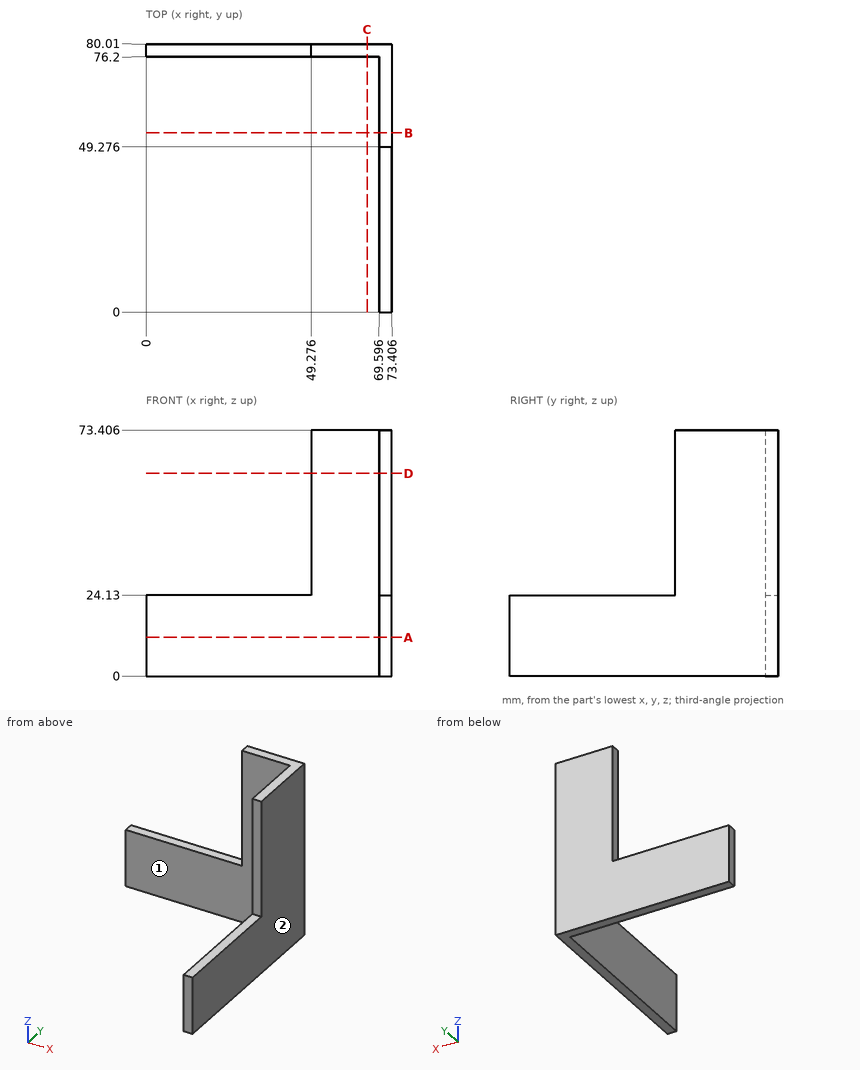
Can you work these out from the drawing? Everything is in mm from the part's minimum corner. A direction names the side the tool comes from. Coordinates: 2 decimals unless noted, no trailing zeros. Loops run counter-clockwise (first coordinate to the right, second up) from the corner with the lowest first, then second, coordinate; pieces in that order, holes last.
1) Will these pins go through, and if not, where does the flat tip stop? pin 1 Ø1.1 at (x, z) = (71.5, 37) entering from -Y; pin 2 Ø1.9 at (x, y) = (28, 78.5) entering from +Z; pin 3 Ø4 at (y, z) = (8.5, 17.5) entering from -X.
Reported:
pin 1: stops at y = 49.28
pin 2: stops at z = 24.13
pin 3: stops at x = 69.6
2) Imagine slicing it at C-C (x = 66). List the corners of the cut face in (y, z) for me, and give its area (3 significant figures).
Reported:
outline: (76.2, 0) - (80.01, 0) - (80.01, 73.41) - (76.2, 73.41) - close
area: 280 mm2
3) Imagine slicing it at B-B (y = 53.5). List the corners of the cut face in (x, z) for me.
Reported:
outline: (69.6, 0) - (73.41, 0) - (73.41, 73.41) - (69.6, 73.41) - close
4) Which directions (+Z, -Z, +X, -X, +Y, -Y) give clear straight access to the entire face, cutting with the end or side of a thin tool? Please do the marked faces 1 and 2.
Reported:
face 1: +Z, -Z, -X, -Y
face 2: +Z, -Z, +X, +Y, -Y
5) Imagine slicing it at A-A (z = 11.5). List the corners of the cut face in (x, y) for me, and give its area (3 significant figures).
Reported:
outline: (0, 76.2) - (69.6, 76.2) - (69.6, 0) - (73.41, 0) - (73.41, 80.01) - (0, 80.01) - close
area: 570 mm2
6) Please list where these lines run through material, in increasing order: line 1 along X through (y, z) = (56.5, 69.5); line 2 along Y through (x, z) = (36.5, 3).
Reported:
line 1: x = 69.6 to 73.41
line 2: y = 76.2 to 80.01
7) Imagine slicing it at D-D (z = 60.5). List the corners of the cut face in (x, y) for me, and give its area (3 significant figures).
Reported:
outline: (49.28, 76.2) - (69.6, 76.2) - (69.6, 49.28) - (73.41, 49.28) - (73.41, 80.01) - (49.28, 80.01) - close
area: 195 mm2
